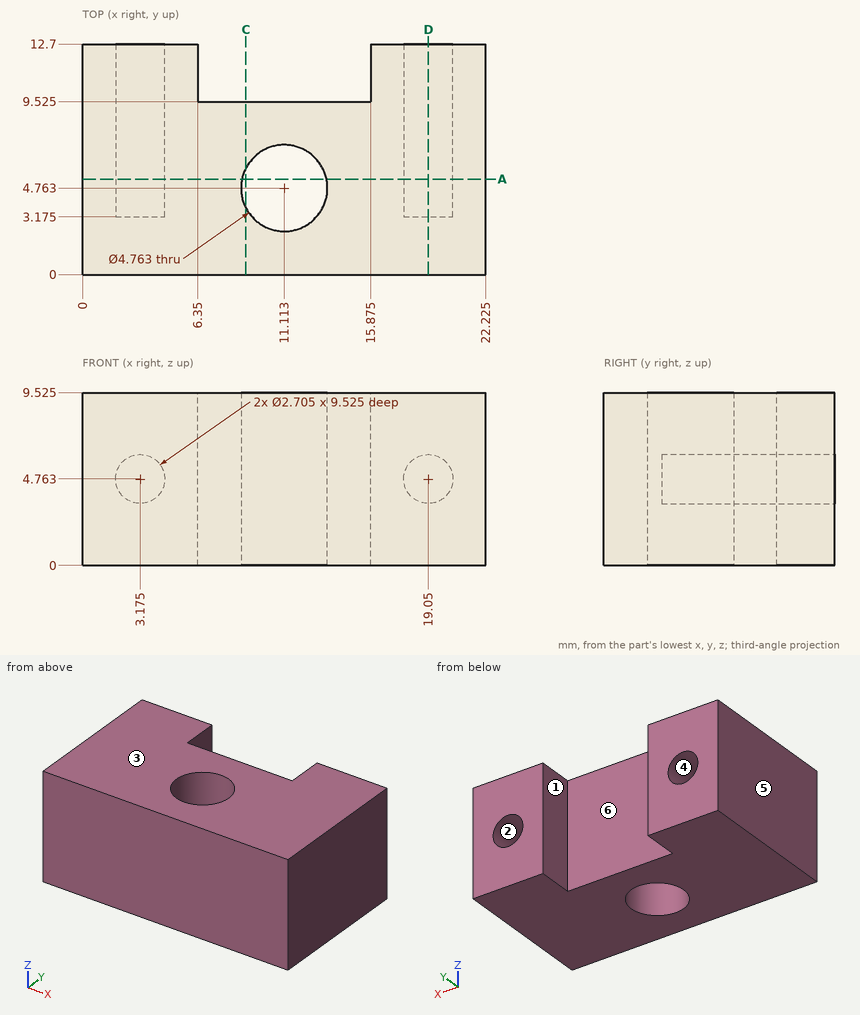
Design review of the part shown in the three views and the two pictorial views. Dimensions are in mm from the part's minimum x, y and z. A direction names the side the tool comes from. Coordinates: 2 decimals unless noted, no trailing zeros. Write each loop counter-clockwise with the first axis right and the second up, starting at its lowest first coordinate (ties: lowest second). Pieces come first, ordered by that corner, then holes.
(1) Tool access review of the marked faces 4, 5 and 6: name each direction out of +Z, -Z, +X, -X, +Y, -Y from which nothing blocks a thin tool from reaching the whole face with its end or side.
(2) Add section C-C on x = 9. Give the boundary of the cut face in (y, z) (1 decimal).
(3) The part is to be moulded in two halves that separate along Z. For the marked faces 1, 2 and 3, say which applies: +Z half, -Z half, draft (parallel to the pull), parting line (faces both ways), or undercut.
(4) Wall thickness on probe 1 along Z at (x, y) = (19.05, 10.5) (1 decimal); probe 2 along X at (y, z) = (5, 4.5) (1 decimal); probe 3 along Y at (x, z) = (15, 7) (1 decimal): over which ranges is each line inside the solid? List them lowest first.
(5) Add section D-D on x = 19.05. Give the boundary of the cut face in (y, z) (1 decimal).
(6) Add section A-A on y = 5.25. Count the separate pieces of the cut face and the enclosed holes in it, then the cut area to 3 significant figures.
Answer sheet:
1. face 4: +Y
1. face 5: +Z, -Z, -X, +Y, -Y
1. face 6: +Z, -Z, +Y
2. outline: (0, 0) - (3.7, 0) - (3.7, 9.5) - (0, 9.5) - close; (5.9, 0) - (9.5, 0) - (9.5, 9.5) - (5.9, 9.5) - close
3. face 1: draft
3. face 2: undercut
3. face 3: +Z half
4. probe 1: z = 0 to 3.4, 6.1 to 9.5
4. probe 2: x = 0 to 1.8, 4.5 to 8.7, 13.5 to 17.7, 20.4 to 22.2
4. probe 3: y = 0 to 9.5
5. outline: (0, 0) - (12.7, 0) - (12.7, 3.4) - (3.2, 3.4) - (3.2, 6.1) - (12.7, 6.1) - (12.7, 9.5) - (0, 9.5) - close
6. separate pieces: 2
6. enclosed holes: 2
6. area: 156 mm2
